The listing builds one solid part. Answer for the finished solid, in the listing's coordinates (mm). A direction names the side the tool comes from. Round coordinates to 2 decimals unless told otherwise and drop trailing zeros. Loops run counter-clockwise (first coordinate to the right, second up) from the corner with the lowest first, then second, coordinate; pieces in that order, holes last. Notation, with made-up numbers: M 9,57 L 54,57 A24 cw 54,90 Z; hole C -10,50 d11. An arc over 180 degrees is marked long. Answer as a JSON object with one key per item and string values.
```python
from build123d import *

# Parameters (mm, degrees)
SKETCH1_W                 = 508
SKETCH1_H                 = 381
BOSS_EXTRUDE1_DEPTH       = 63.5
FILLET4_R                 = 12.7
FILLET5_R                 = 12.7
FILLET6_R                 = 12.7
FILLET7_R                 = 12.7
FILLET8_R                 = 12.7
FILLET9_R                 = 12.7
SKETCH2_W                 = 185.582579438
SKETCH2_H                 = 101.6
BOSS_EXTRUDE2_DEPTH       = 406.4
SKETCH26_W                = 101.6
SKETCH26_H                = 101.6
BOSS_EXTRUDE16_DEPTH      = 558.8
SKETCH28_W                = 101.849960699
SKETCH28_H                = 50.8
CUT_EXTRUDE8_DEPTH        = 127
SKETCH29_W                = 124.46
SKETCH29_H                = 50.8
BOSS_EXTRUDE18_DEPTH      = 88.9
FILLET10_R                = 12.7
BOSS_EXTRUDE21_DEPTH      = 18.796
BOSS_EXTRUDE21_DEPTH_BACK = 73.66
SKETCH31_R                = 17.78
BOSS_EXTRUDE22_DEPTH      = 14.986
BOSS_EXTRUDE22_DEPTH_BACK = 71.374
SKETCH32_R                = 19.05
SKETCH33_R                = 30.48
CUT_EXTRUDE10_DEPTH       = 71.374
SCALE1_SCALE              = 1.5


with BuildPart() as part:
    # Sketch1 → Boss-Extrude1 (new body)
    with BuildSketch(Plane(origin=(0, 0, 0), x_dir=(1, 0, 0), z_dir=(0, 1, 0))):
        with Locations((254, 190.5)):
            Rectangle(SKETCH1_W, SKETCH1_H)
    extrude(amount=BOSS_EXTRUDE1_DEPTH)

    # Fillet4
    fillet4_edges = [part.edges().sort_by_distance(p)[0] for p in [
        (508, 31.75, 0),
    ]]
    fillet(fillet4_edges, radius=FILLET4_R)

    # Fillet5
    fillet5_edges = [part.edges().sort_by_distance(p)[0] for p in [
        (508, 31.75, -381),
    ]]
    fillet(fillet5_edges, radius=FILLET5_R)

    # Fillet6
    fillet6_edges = [part.edges().sort_by_distance(p)[0] for p in [
        (0, 31.75, -381),
    ]]
    fillet(fillet6_edges, radius=FILLET6_R)

    # Fillet7
    fillet7_edges = [part.edges().sort_by_distance(p)[0] for p in [
        (0, 31.75, 0),
    ]]
    fillet(fillet7_edges, radius=FILLET7_R)

    # Fillet8
    fillet8_edges = [part.edges().sort_by_distance(p)[0] for p in [
        (508, 0, -190.5),
        (504.280256121, 0, -3.719743879),
        (254, 0, -381),
        (504.280256121, 0, -377.280256121),
        (0, 0, -190.5),
        (3.719743879, 0, -377.280256121),
        (254, 0, 0),
        (3.719743879, 0, -3.719743879),
    ]]
    fillet(fillet8_edges, radius=FILLET8_R)

    # Fillet9
    fillet9_edges = [part.edges().sort_by_distance(p)[0] for p in [
        (508, 63.5, -190.5),
        (504.280256121, 63.5, -3.719743879),
        (254, 63.5, -381),
        (504.280256121, 63.5, -377.280256121),
        (0, 63.5, -190.5),
        (3.719743879, 63.5, -377.280256121),
        (254, 63.5, 0),
        (3.719743879, 63.5, -3.719743879),
    ]]
    fillet(fillet9_edges, radius=FILLET9_R)

    # Sketch2 → Boss-Extrude2 (add)
    with BuildSketch(Plane(origin=(0, 63.5, 0), x_dir=(1, 0, 0), z_dir=(0, 1, 0))):
        with Locations((212.008710281, 190.5)):
            Rectangle(SKETCH2_W, SKETCH2_H)
    extrude(amount=BOSS_EXTRUDE2_DEPTH)

    # Sketch26 → Boss-Extrude16 (add)
    with BuildSketch(Plane.ZY.offset(-119.217420562)):
        with Locations((-190.5, 520.7)):
            Rectangle(SKETCH26_W, SKETCH26_H)
    extrude(amount=-BOSS_EXTRUDE16_DEPTH)

    # Sketch28 → Cut-Extrude8 (cut)
    with BuildSketch(Plane(origin=(680.557420562, 0, 0), x_dir=(0, 0, -1), z_dir=(1, 0, 0))):
        with Locations((190.588941682, 550.48771611)):
            Rectangle(SKETCH28_W, SKETCH28_H)
    extrude(amount=-CUT_EXTRUDE8_DEPTH, mode=Mode.SUBTRACT)

    # Sketch29 → Boss-Extrude18 (add)
    with BuildSketch(Plane(origin=(0, 525.08771611, 0), x_dir=(1, 0, 0), z_dir=(0, 1, 0))):
        with Locations((615.787420562, 190.5)):
            Rectangle(SKETCH29_W, SKETCH29_H)
    extrude(amount=BOSS_EXTRUDE18_DEPTH)

    # Fillet10
    fillet10_edges = [part.edges().sort_by_distance(p)[0] for p in [
        (119.217420562, 571.5, -190.5),
    ]]
    fillet(fillet10_edges, radius=FILLET10_R)

    # Sketch31 → Boss-Extrude21 (add, two sides: drawn at the far end of the back side and taken through both)
    with BuildSketch(Plane(origin=(0, 0, -218.44), x_dir=(-1, 0, 0), z_dir=(0, 0, -1)).offset(-BOSS_EXTRUDE21_DEPTH_BACK)):
        with Locations((-640.580859251, 525.041927268)):
            Circle(SKETCH31_R)
    extrude(amount=BOSS_EXTRUDE21_DEPTH + BOSS_EXTRUDE21_DEPTH_BACK)

    # Sketch32 → Boss-Extrude22 (add, two sides: drawn at the far end of the back side and taken through both)
    with BuildSketch(Plane(origin=(0, 0, -218.44), x_dir=(-1, 0, 0), z_dir=(0, 0, -1)).offset(-BOSS_EXTRUDE22_DEPTH_BACK)):
        with Locations((-601.906085303, 524.903929641)):
            Circle(SKETCH32_R)
    extrude(amount=BOSS_EXTRUDE22_DEPTH + BOSS_EXTRUDE22_DEPTH_BACK)

    # Sketch33 → Cut-Extrude10 (cut)
    with BuildSketch(Plane(origin=(0, 0, -218.44), x_dir=(-1, 0, 0), z_dir=(0, 0, -1))):
        with Locations((-621.346482392, 580.790680071)):
            Circle(SKETCH33_R)
    extrude(amount=-CUT_EXTRUDE10_DEPTH, mode=Mode.SUBTRACT)


with BuildPart() as part_1:
    # Scale1: scaled about (272.242227358, 210.761068124, -190.500428021)
    add(part.part.scale(SCALE1_SCALE).moved(Location((-136.121113679, -105.380534062, 95.250214011))))


solid = part_1.part
```
Item 1: The part is cut by section B-B (z = -182.5). Give the vertices of the cut face in (x, y), then the cut area to 3 significant figures.
Values follow:
{"outline": "M -136.12,-86.33 A19.05 ccw -117.07,-105.38 L 606.83,-105.38 A19.05 ccw 625.88,-86.33 L 625.88,-29.18 A19.05 ccw 606.83,-10.13 L 321.08,-10.13 L 321.08,599.47 L 880.91,599.47 L 880.91,815.6 L 694.22,815.6 L 694.22,751.87 L 61.76,751.87 A19.05 ccw 42.71,732.82 L 42.71,-10.13 L -117.07,-10.13 A19.05 ccw -136.12,-29.18 Z; hole C 795.9,765.81 d91.44", "area": "375,000 mm^2"}
Item 2: The part is cut by section A-A (x = 568). Give the vertices of the cut face in (y, z), then the cut area to 3 significant figures.
Values follow:
{"outline": "M -105.38,-457.2 A19.05 ccw -86.33,-476.25 L -29.18,-476.25 A19.05 ccw -10.13,-457.2 L -10.13,76.2 A19.05 ccw -29.18,95.25 L -86.33,95.25 A19.05 ccw -105.38,76.2 Z; M 599.47,-266.7 L 751.87,-266.7 L 751.87,-114.3 L 599.47,-114.3 Z", "area": "77,300 mm^2"}
Item 3: Determine the mould class of faces 1 (the face through (-136.121, -58, -187)), 2 (the face through (767, 693, -254.889)), 3 (the face through (240, -105.381, -194)) for opening direction X: released by +X, released by -X, zero draft, split by the parting line, or undercut.
Values follow:
{"face 1": "released by -X", "face 2": "undercut", "face 3": "zero draft"}
Item 4: Straight lines are drawn through the part: line 1 (Y direction, x = 408.5, z = -169); line 2 (X direction, y = 613.5, z = -254); line 3 (Y direction, x = 197.5, z = -310.5). For each, find the intervals that lie inside material, in ascending order.
Values follow:
{"line 1": "-105.38 to -10.13, 599.47 to 751.87", "line 2": "42.71 to 880.91", "line 3": "-105.38 to -10.13"}
Item 5: The part is cut by section D-D (y = -47.5). Give the vertices of the cut face in (x, z).
Values follow:
{"outline": "M -136.12,-457.2 A19.05 ccw -117.07,-476.25 L 606.83,-476.25 A19.05 ccw 625.88,-457.2 L 625.88,76.2 A19.05 ccw 606.83,95.25 L -117.07,95.25 A19.05 ccw -136.12,76.2 Z"}
Item 6: Flat-ended cylindrical pins translate along their axes: P1, Ø22.5, axis at x = 756, y = 701, coming from the -Z side; P2, Ø19, axis at y = 797.5, z = -203.5, coming from the -X side (3 decimals); P3, Ø6, axis at y = 664, z = -258, coming from the -X side (3 decimals). Find the tip coordinate at first contact, or state that the pin passes through.
Values follow:
{"P1": "z = -254.89", "P2": "x = 694.215", "P3": "x = 42.705"}
Item 7: The part is cut by section C-C (x = -35). Give the vertices of the cut face in (y, z).
Values follow:
{"outline": "M -105.38,-457.2 A19.05 ccw -86.33,-476.25 L -29.18,-476.25 A19.05 ccw -10.13,-457.2 L -10.13,76.2 A19.05 ccw -29.18,95.25 L -86.33,95.25 A19.05 ccw -105.38,76.2 Z"}
Item 8: Which of the six approach directions +Z, -Z, +X, -X, +Y, -Y give full straight-line access (tool end or side, diameter ignored) to faces 4 (the face through (768, 682.251, -256)), 5 (the face through (825, 693, -121.92)), 6 (the face through (824.165, 708.846, -136.946)), 7 (the face through (270, 450, -266.7)), 8 (the face through (694.215, 783, -190))?
Values follow:
{"face 4": "-Z, +Y", "face 5": "+Z, +X, +Y", "face 6": "+Z, +Y", "face 7": "-Z, +X, -X, +Y", "face 8": "+Z, -Z, -X, +Y"}
